```python
from build123d import *

# Parameters (mm, degrees)
PAD_DEPTH        = 19.05
FILLET_R         = 1.27
HOLE_D           = 4.1
HOLE_DEPTH       = 14.986
HOLE_CSINK_D     = 5.3594
HOLE_CSINK_ANGLE = 82
HOLE_TIPS_R      = 2.05
SKETCH002_R      = 63.5
POCKET_DEPTH     = 9.525
POCKET001_DEPTH  = 3.175
POCKET002_DEPTH  = 16.51
FILLET001_R      = 2.54
CHAMFER_SIZE     = 0.254


with BuildPart() as part:
    # Sketch → Pad (new body)
    with BuildSketch(Plane.XY):
        Polygon((-29.21, 0), (29.21, 0), (0, 50.8), align=None)
    extrude(amount=PAD_DEPTH)

    # Fillet
    fillet_edges = [part.edges().sort_by_distance(p)[0] for p in [
        (-29.21, 0, 9.525),
        (29.21, 0, 9.525),
        (0, 50.8, 9.525),
    ]]
    fillet(fillet_edges, radius=FILLET_R)

    # Hole
    with Locations(Plane.XY.offset(19.05)):
        with Locations((0, 41.5798), (21.0312, 4.8006), (-21.0312, 4.8006)):
            CounterSinkHole(HOLE_D / 2, HOLE_CSINK_D / 2, depth=HOLE_DEPTH, counter_sink_angle=HOLE_CSINK_ANGLE)

    # Hole tips → Hole tip 1 section 0
    with BuildSketch(Plane.XY.offset(4.064), mode=Mode.PRIVATE) as hole_tip_1_s0:
        with Locations((0, 41.5798)):
            Circle(HOLE_TIPS_R)
    loft([hole_tip_1_s0.sketch, Vertex(0, 41.5798, 2.832236)], mode=Mode.SUBTRACT)

    # Hole tips → Hole tip 2 section 0
    with BuildSketch(Plane.XY.offset(4.064), mode=Mode.PRIVATE) as hole_tip_2_s0:
        with Locations((21.0312, 4.8006)):
            Circle(HOLE_TIPS_R)
    loft([hole_tip_2_s0.sketch, Vertex(21.0312, 4.8006, 2.832236)], mode=Mode.SUBTRACT)

    # Hole tips → Hole tip 3 section 0
    with BuildSketch(Plane.XY.offset(4.064), mode=Mode.PRIVATE) as hole_tip_3_s0:
        with Locations((-21.0312, 4.8006)):
            Circle(HOLE_TIPS_R)
    loft([hole_tip_3_s0.sketch, Vertex(-21.0312, 4.8006, 2.832236)], mode=Mode.SUBTRACT)

    # Sketch002 (on Face5 of Hole) → Pocket (cut)
    with BuildSketch(Plane.XY.offset(19.05)):
        Circle(SKETCH002_R)
        with BuildLine():
            Line((-25.198579, 7.183604), (-4.167379, 43.962804))
            ThreePointArc((4.167379, 43.962804), (0, 46.3804), (-4.167379, 43.962804))
            Line((4.167379, 43.962804), (25.198579, 7.183604))
            ThreePointArc((21.0312, 0), (25.183646, 2.391668), (25.198579, 7.183604))
            Line((21.0312, 0), (-21.0312, 0))
            ThreePointArc((-25.198579, 7.183604), (-25.183646, 2.391668), (-21.0312, 0))
        make_face(mode=Mode.SUBTRACT)
    extrude(amount=-POCKET_DEPTH, mode=Mode.SUBTRACT)

    # Sketch003 (on Face13 of Pocket) → Pocket001 (cut)
    with BuildSketch(Plane.XY.offset(9.525)):
        with BuildLine():
            ThreePointArc((-62.664993, -0.912406), (-12.437232, 24.117556), (-15.907518, 80.129021))
            Line((-15.907518, 80.129021), (-62.664993, -0.912406))
        make_face()
        with BuildLine():
            ThreePointArc((15.907518, 80.129021), (12.437232, 24.117556), (62.664993, -0.912406))
            Line((15.907518, 80.129021), (62.664993, -0.912406))
        make_face()
        with BuildLine():
            ThreePointArc((46.781338, -28.414351), (0, 2.582963), (-46.781338, -28.414351))
            Line((46.781338, -28.414351), (-46.781338, -28.414351))
        make_face()
    extrude(amount=POCKET001_DEPTH, mode=Mode.SUBTRACT)

    # Sketch004 (on Face6 of Pocket001) → Pocket002 (cut)
    with BuildSketch(Plane.XY.offset(19.05)):
        with BuildLine():
            Line((-13.272642, 4.4196), (13.272642, 4.4196))
            ThreePointArc((13.272642, 4.4196), (17.430084, 6.8199), (17.430084, 11.6205))
            Line((17.430084, 11.6205), (4.157442, 34.609391))
            ThreePointArc((4.157442, 34.609391), (0, 37.009691), (-4.157442, 34.609391))
            Line((-4.157442, 34.609391), (-17.430084, 11.6205))
            ThreePointArc((-17.430084, 11.6205), (-17.430084, 6.8199), (-13.272642, 4.4196))
        make_face()
    extrude(amount=-POCKET002_DEPTH, mode=Mode.SUBTRACT)

    # Fillet001
    fillet001_edges = [part.edges().sort_by_distance(p)[0] for p in [
        (-3.293151, 45.072781, 14.2875),
        (3.293151, 45.072781, 14.2875),
        (25.597076, 6.283346, 14.2875),
        (-25.597076, 6.283346, 14.2875),
    ]]
    fillet(fillet001_edges, radius=FILLET001_R)

    # Chamfer
    chamfer_edges = [part.edges().sort_by_distance(p)[0] for p in [
        (-10.793763, 23.114945, 19.05),
        (-14.477962, 25.620935, 19.05),
        (0, 0, 0),
    ]]
    chamfer(chamfer_edges, length=CHAMFER_SIZE)


solid = part.part
```
Check sheet for the modelled part. Datum: model origin and axes. Units: mm. A direction names the side the tool comes from. Coordinates: 2 decimals unless noted, no trailing zeros. Order: outer loops, then holes, each group sorted by start corner. A loop starts at its lowest first (then second) coordinate and runs counter-clockwise, first axis right, second up. Notation, with made-up numbers: M 28,-16.5 L 78,-16.5 A30 cw 78,8.5 Z; hole C -39.75,2.25 d10. An arc over 180 degrees is marked long. Write each question's results on one line, items separated by ' | '. Start each with the question number.
1. Cross-section at A-A on z = 16.5. Record the cut outline in (x, y).
2. Cross-section at B-B on y = 15. Record the cut outline in (x, z) (3 decimals).
3. Go/stop test with flat-tipped pins: P1, Ø5, axis at y = 6.5, z = 16.5, coming from the +X side; P2, Ø5, axis at y = 18, z = 5.5, coming from the -X side; P3, Ø16.5, axis at x = -2, y = 21, coming from the +Z side. Record where each tip stops, or that it passes through.
4. Material ranges on probe 1 along Y at (x, z) = (-1, 5.5); probe 2 along X at (y, z) = (6.5, 15.5); probe 3 along Y at (x, z) = (16.5, 16.75), recorded low to high.
5. Cross-section at C-C on z = 8. Record the cut outline in (x, y), and give its area (3 significant figures).
6. Access from +Z, -Z, +X, -X, +Y, -Y to the whole of each face (thin tool, end or side, straight path). Record for faces 4 (the face through (-12.51, 23.99, 11.09)), 5 (the face through (-17.465, 6.881, 10.782)), 6 (the face through (0.228, 2.582, 11.09)).
7. Mould release check, pull along Z, two halves, no side actions. Record for faces 1 (the face through (20.7, 4.81, 3.03)), 2 (the face through (12.288, 24.377, 11.09)), 3 (the face through (-28.011, 0.713, 0.125)): +Z half, -Z half, draft (parallel to the pull), parting line (faces both ways), or undercut.
Checks:
1) outline: M -25.72,5.84 A4.8 ccw -21.03,0 L 21.03,0 A4.8 ccw 25.72,5.84 A2.54 ccw 25.44,6.56 L 3.52,44.69 A2.54 ccw 2.79,45.49 A4.8 ccw -2.79,45.49 A2.54 ccw -3.52,44.69 L -25.44,6.56 A2.54 ccw Z; hole C -21.03,4.8 d4.1; hole M -17.43,11.62 A4.8 ccw -13.27,4.42 L 13.27,4.42 A4.8 ccw 17.43,11.62 L 4.16,34.61 A4.8 ccw -4.16,34.61 Z; hole C 0,41.58 d4.1; hole C 21.03,4.8 d4.1
2) outline: M -20.585,0.254 L -20.292,0 L 20.292,0 L 20.585,0.254 L 20.585,9.525 L 19.155,9.525 L 19.155,12.7 L 20.585,12.7 L 20.585,18.796 L 20.292,19.05 L 15.772,19.05 L 15.479,18.796 L 15.479,2.54 L -15.479,2.54 L -15.479,18.796 L -15.772,19.05 L -20.292,19.05 L -20.585,18.796 L -20.585,12.7 L -19.155,12.7 L -19.155,9.525 L -20.585,9.525 Z
3) P1: stops at x = 25.83 | P2: stops at x = -20.3 | P3: stops at z = 2.54
4) probe 1: y = 0 to 4.42, 36.9 to 39.79, 43.37 to 49.04 | probe 2: x = -25.47 to -22.18, -19.88 to -17.23, 17.23 to 19.88, 22.18 to 25.47 | probe 3: y = 0 to 5.67, 13.23 to 22.1
5) outline: M -28.12,1.9 A1.27 ccw -27.01,0 L 27.01,0 A1.27 ccw 28.12,1.9 L 1.1,48.89 A1.27 ccw -1.1,48.89 Z; hole C -21.03,4.8 d4.1; hole M -17.43,11.62 A4.8 ccw -13.27,4.42 L 13.27,4.42 A4.8 ccw 17.43,11.62 L 4.16,34.61 A4.8 ccw -4.16,34.61 Z; hole C 0,41.58 d4.1; hole C 21.03,4.8 d4.1 | area: 681 mm²
6) face 4: -X, +Y | face 5: +Z | face 6: -Y
7) face 1: +Z half | face 2: undercut | face 3: -Z half
